Part model, mm, in its own coordinate system. Coordinates: 2 decimals unless noted, no trailing zeros. Order: outer loops, then holes, each group sorted by start corner. A loop starts at its lowest first (then second) coordinate and runs counter-clockwise, first axis right, second up.
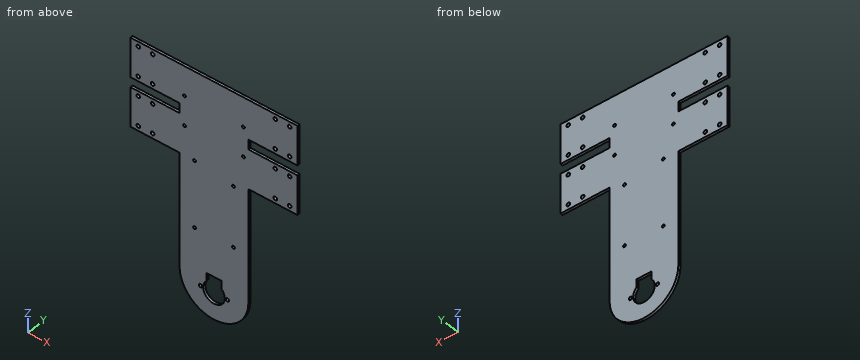
from build123d import *

# Parameters (mm, degrees)
SKETCH1_W           = 63.5
SKETCH1_H           = 50.8
BOSS_EXTRUDE1_DEPTH = 3.175
SKETCH2_R           = 1.80975
SKETCH2_R_2         = 2.159
CUT_EXTRUDE1_DEPTH  = 4.175
SKETCH3_R           = 2.3495
CUT_EXTRUDE2_DEPTH  = 4.175


with BuildPart() as part:
    # Sketch1 → Boss-Extrude1 (new body)
    with BuildSketch(Plane(origin=(0, 0, 0), x_dir=(1, 0, 0), z_dir=(0, 1, 0))):
        with Locations((-76.2, -63.5)):
            Rectangle(SKETCH1_W, SKETCH1_H)
        with BuildLine():
            ThreePointArc((44.45, 107.95), (0, 152.4), (-44.45, 107.95))
            Line((-44.45, 107.95), (-44.45, -38.1))
            Line((-44.45, -38.1), (-44.45, -88.9))
            Line((-44.45, -88.9), (-44.45, -101.6))
            Line((-44.45, -101.6), (-44.45, -152.4))
            Line((-44.45, -152.4), (44.45, -152.4))
            Line((44.45, -152.4), (44.45, -101.6))
            Line((44.45, -101.6), (44.45, -88.9))
            Line((44.45, -88.9), (44.45, -38.1))
            Line((44.45, -38.1), (44.45, 107.95))
        make_face()
        with Locations((76.2, -63.5)):
            Rectangle(SKETCH1_W, SKETCH1_H)
        with Locations((76.2, -127)):
            Rectangle(SKETCH1_W, SKETCH1_H)
        with Locations((-76.2, -127)):
            Rectangle(SKETCH1_W, SKETCH1_H)
    extrude(amount=BOSS_EXTRUDE1_DEPTH)

    # Sketch2 → Cut-Extrude1 (cut, through all)
    with BuildSketch(Plane(origin=(0, 3.175, 0), x_dir=(1, 0, 0), z_dir=(0, 1, 0))):
        with Locations((-38.1, -76.2)):
            Circle(SKETCH2_R)
        with Locations((38.1, -76.2)):
            Circle(SKETCH2_R)
        with Locations((-38.1, -114.3)):
            Circle(SKETCH2_R)
        with Locations((38.1, -114.3)):
            Circle(SKETCH2_R)
        with Locations((-25.14473, 47.72914)):
            Circle(SKETCH2_R)
        with Locations((25.14473, 46.58614)):
            Circle(SKETCH2_R)
        with Locations((25.14473, -31.56966)):
            Circle(SKETCH2_R)
        with Locations((-25.14473, -38.1)):
            Circle(SKETCH2_R)
        with Locations((-17.526, 118.11)):
            Circle(SKETCH2_R_2)
        with Locations((17.526, 118.11)):
            Circle(SKETCH2_R_2)
        with BuildLine():
            Line((-9.525, 107.890642143), (-9.525, 97.730642143))
            Line((-9.525, 97.730642143), (9.525, 97.730642143))
            Line((9.525, 97.730642143), (9.525, 107.890642143))
            ThreePointArc((9.525, 107.890642143), (0, 132.08), (-9.525, 107.890642143))
        make_face()
    extrude(amount=-CUT_EXTRUDE1_DEPTH, mode=Mode.SUBTRACT)

    # Sketch3 → Cut-Extrude2 (cut, through all)
    with BuildSketch(Plane(origin=(0, 3.175, 0), x_dir=(1, 0, 0), z_dir=(0, 1, 0))):
        with Locations((-97.8535, -44.45)):
            Circle(SKETCH3_R)
        with Locations((-79.3115, -44.45)):
            Circle(SKETCH3_R)
        with Locations((-97.8535, -82.55)):
            Circle(SKETCH3_R)
        with Locations((-79.3115, -82.55)):
            Circle(SKETCH3_R)
        with Locations((-79.3115, -107.95)):
            Circle(SKETCH3_R)
        with Locations((-97.8535, -107.95)):
            Circle(SKETCH3_R)
        with Locations((-79.3115, -146.05)):
            Circle(SKETCH3_R)
        with Locations((-97.8535, -146.05)):
            Circle(SKETCH3_R)
        with Locations((97.8535, -146.05)):
            Circle(SKETCH3_R)
        with Locations((79.3115, -146.05)):
            Circle(SKETCH3_R)
        with Locations((97.8535, -107.95)):
            Circle(SKETCH3_R)
        with Locations((79.3115, -107.95)):
            Circle(SKETCH3_R)
        with Locations((79.3115, -82.55)):
            Circle(SKETCH3_R)
        with Locations((97.8535, -82.55)):
            Circle(SKETCH3_R)
        with Locations((79.3115, -44.45)):
            Circle(SKETCH3_R)
        with Locations((97.8535, -44.45)):
            Circle(SKETCH3_R)
    extrude(amount=-CUT_EXTRUDE2_DEPTH, mode=Mode.SUBTRACT)


solid = part.part
Q1. Pin check, flat tips, straight feed: pin 1 Ø1.6 at (y, z) = (1, -38) entering from +X; pin 2 Ø1 at (x, y) = (-78.5, 1.5) entering from -Z. Stop position of each tip, or through.
Results list:
pin 1: stops at x = 44.45
pin 2: stops at z = 38.1
Q2. Cut at A-A on x = 0. Write the cut outline in (y, z) (3 decimals).
Results list:
outline: (0, -152.4) - (3.175, -152.4) - (3.175, -132.08) - (0, -132.08) - close; (0, -97.731) - (3.175, -97.731) - (3.175, 152.4) - (0, 152.4) - close
Q3. Cut at B-B on z = -5.5. Write the cut outline in (x, y) (3 decimals).
Results list:
outline: (-44.45, 0) - (44.45, 0) - (44.45, 3.175) - (-44.45, 3.175) - close
Q4. Cut at C-C on y = 2.35. Count the separate pieces of the cut face and the enclosed holes in it, and give its area (3 significant figures).
Results list:
separate pieces: 1
enclosed holes: 27
area: 38,000 mm2
Q5. Wall check: line 1 along X through (y, z) = (0.85, 107.95); line 2 along X through (y, z) = (1.8, 114.3); line 3 along Z through (x, y) = (-49, 0.8). Give the ranges that are in metal, low to high.
Results list:
line 1: x = -107.95 to -100.2, -95.5 to -81.66, -76.96 to 76.96, 81.66 to 95.5, 100.2 to 107.95
line 2: x = -107.95 to -39.91, -36.29 to 36.29, 39.91 to 107.95
line 3: z = 38.1 to 88.9, 101.6 to 152.4
